Can you work these out from the drawing? Everything is in mm from the part's minimum corner. A direction names the side the tool comes from. Give positions to 0.01 mm unless a question says otherwise; leave off trailing zeros. Write each loop counter-clockwise with the first axis right and the second up, starting at its lowest first coordinate (ties: lowest second). Pieces come first, ordered by that corner, then holes. Notation, with made-up numbers: (67, 36.5) -> (103, 36.5) arc R31 ccw to (103, 60.5) -> close; hole circle Ø5 at (30, 61). An arc over 180 degrees is marked (long way). Use one line per item in the form item = value.
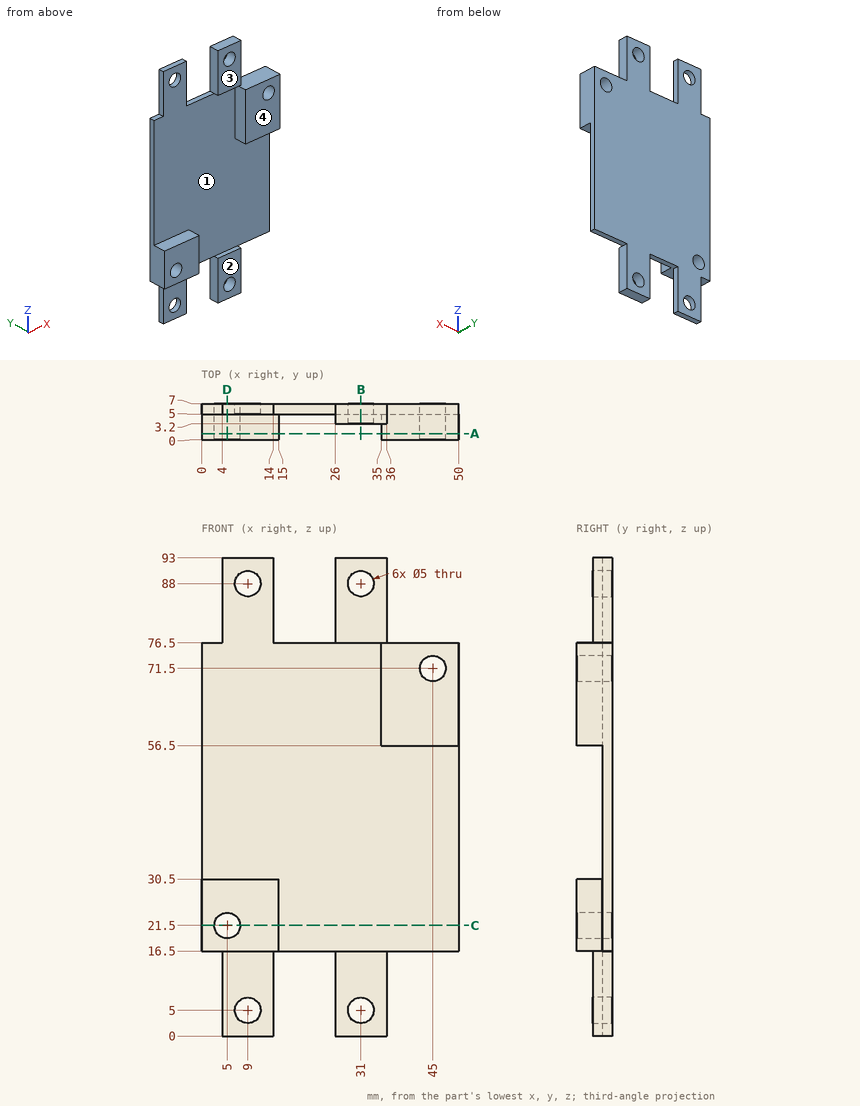
Q1. I want a section at A-A, the plane y = 1.25. Write out the boundary of the cut face in (x, z).
Result set:
outline = (0, 16.5) -> (15, 16.5) -> (15, 30.5) -> (0, 30.5) -> close; (35, 56.5) -> (50, 56.5) -> (50, 76.5) -> (35, 76.5) -> close; hole circle Ø5 at (5, 21.5); hole circle Ø5 at (45, 71.5)
Q2. Which directions (+Z, -Z, +X, -X, +Y, -Y) give clear straight access to the entire face, cutting with the end or side of a thin tool? Please do the marked faces 3 and 4.
Result set:
face_3 = +Z, +X, -X, -Y
face_4 = +Z, -Z, +X, -X, -Y
Q3. I want a section at C-C, the plane z = 21.5. Write out the boundary of the cut face in (x, y), and give its area (3 significant figures).
Result set:
outline = (0, 0) -> (2.5, 0) -> (2.5, 7) -> (0, 7) -> close; (7.5, 0) -> (15, 0) -> (15, 5) -> (50, 5) -> (50, 7) -> (7.5, 7) -> close
area = 140 mm2
Q4. Will these pins go through, and if not, where does the flat tip stop? pin 1 Ø2.5 at (x, y) = (40.5, 3.5) entering from -Z; pin 2 Ø3 at (x, y) = (13.5, 2) entering from -Z; pin 3 Ø1 at (x, y) = (28, 1) entering from +Z; pin 4 Ø1.6 at (x, y) = (1, 5.5) entering from +Z.
Result set:
pin_1 = 56.5
pin_2 = 16.5
pin_3 = through
pin_4 = 76.5
Q5. If we mould it in two halves opening along Z, with no side actions, what happens to the marked faces 1 and 2? For each: +Z half, -Z half, draft (parallel to the pull), parting line (faces both ways), or undercut.
Result set:
face_1 = undercut
face_2 = draft
Q6. If I drill on line 1 along X through (y, z) = (4.75, 21.5); line 2 along X through (y, z) = (2.5, 71.5); line 3 along Y through (x, z) = (32.5, 72), over which ranges is the centre line in solid material (lowest first)? Write a range as from..to.
Result set:
line_1 = 0..2.5, 7.5..15
line_2 = 35..42.5, 47.5..50
line_3 = 5..7
Q7. I want a section at B-B, the plane x = 31. Write out the boundary of the cut face in (y, z).
Result set:
outline = (3.2, 0) -> (7, 0) -> (7, 2.5) -> (3.2, 2.5) -> close; (3.2, 7.5) -> (7, 7.5) -> (7, 85.5) -> (3.2, 85.5) -> (3.2, 76.5) -> (5, 76.5) -> (5, 16.5) -> (3.2, 16.5) -> close; (3.2, 90.5) -> (7, 90.5) -> (7, 93) -> (3.2, 93) -> close
Q8. I want a section at D-D, the plane x = 5. Write out the boundary of the cut face in (y, z).
Result set:
outline = (0, 16.5) -> (5, 16.5) -> (5, 0) -> (7, 0) -> (7, 19) -> (0, 19) -> close; (0, 24) -> (7, 24) -> (7, 93) -> (5, 93) -> (5, 30.5) -> (0, 30.5) -> close
